Could you check a few things on this model? Use its own coordinates, in mm. A direction names the side the tool comes from. Give positions to 0.01 mm unless a question says otherwise; leave off trailing zeros. Write each loop counter-clockwise with the first axis right and the second up, starting at its lowest first coordinate (ties: lowest second). Pieces come first, ordered by that corner, then holes. Notation, with made-up numbers: (71.25, -21.75) -> (91.25, -21.75) arc R17 ccw to (91.25, 0.25) -> close; hole circle Ø8 at (33.25, 12.25). An arc over 180 degrees is marked (long way). Write item = value, one per line. Start each with the question number.
```python
from build123d import *

# Parameters (mm, degrees)
SKETCH_1_W             = 42
SKETCH_1_H             = 10
EXTRUDE_1_DEPTH        = 23.5
CUT_EXTRUDE_1_DEPTH    = 52.720402164
HOLE_WIZARD_M4_2_D     = 3.3
HOLE_WIZARD_M4_2_DEPTH = 10.1
HOLE_WIZARD_M4_2_TIP   = 0.991420021
HOLE_WIZARD_M4_1_D     = 3.3
CHAMFER_4_SIZE         = 12
CUT_EXTRUDE_3_DEPTH    = 34.064331336


with BuildPart() as part:
    # 草图1 → 凸台-拉伸1 (new, symmetric)
    with BuildSketch(Plane(origin=(0, 0, 0), x_dir=(0, 0, -1), z_dir=(1, 0, 0))):
        Rectangle(SKETCH_1_W, SKETCH_1_H)
    extrude(amount=EXTRUDE_1_DEPTH, both=True)

    # 草图2 → 切除-拉伸1 (cut, through all)
    with BuildSketch(Plane(origin=(23.5, 0, 0), x_dir=(0, 0, -1), z_dir=(1, 0, 0))):
        Polygon((21, -5), (11, 5), (21, 5), align=None)
    extrude(amount=-CUT_EXTRUDE_1_DEPTH, mode=Mode.SUBTRACT)

    # M4 螺纹孔2
    with Locations(Plane(origin=(-23.5, -27.863076326, 2.458563873), x_dir=(0, -1, 0), z_dir=(-1, 0, 0))):
        with Locations((-27.863076326, 5.541436127), (-27.863076326, -6.458563873)):
            Hole(HOLE_WIZARD_M4_2_D / 2, depth=HOLE_WIZARD_M4_2_DEPTH)
            with Locations((0, 0, -(HOLE_WIZARD_M4_2_DEPTH + HOLE_WIZARD_M4_2_TIP / 2))):  # 118° drill point
                Cone(0, HOLE_WIZARD_M4_2_D / 2, HOLE_WIZARD_M4_2_TIP, mode=Mode.SUBTRACT)

    # M4 螺纹孔1 (through all)
    with Locations(Plane(origin=(0, -5, 0), x_dir=(-1, 0, 0), z_dir=(0, -1, 0))):
        with Locations((-2.5, 17), (-17.222431864, -8.5), (12.222431864, -8.5)):
            Hole(HOLE_WIZARD_M4_1_D / 2)

    # 倒角4
    chamfer_4_edges = [part.edges().sort_by_distance(p)[0] for p in [
        (23.5, 0, 21),
    ]]
    chamfer(chamfer_4_edges, length=CHAMFER_4_SIZE)

    # 草图8 → 切除-拉伸3 (cut, through all)
    with BuildSketch(Plane.XZ.offset(5)):
        Polygon((23.5, -9), (11.5, -21), (23.5, -21), align=None)
    extrude(amount=-CUT_EXTRUDE_3_DEPTH, mode=Mode.SUBTRACT)


solid = part.part
```
(1) Imagine slicing it at C-C (y = -2.5). Please give me the cut outline in (x, z).
(2) On a 3-axis mill with a long thin cutter (end or side, diameter ignored), from which of +Z, -Z, +X, -X, +Y, -Y can I reach the whole of each face in a straight line? I mean faces 1 (the cylindrical face through (2.1, -2.7, -15.4)), 2 (the cylindrical face through (-18.379, -1.216, 9.115)). Say none if no direction works.
(3) I'm going to push flat-ended pins straight in: pin 1 (2 mm diameter, centred on x = 13, y = 2.5, fed in from -Z); pin 2 (4 mm diameter, centred on y = 2.5, z = -14.5, fed in from +X); pin 3 (5.5 mm diameter, centred on x = 2.5, z = -17, fed in from +Y); pin 4 (2 mm diameter, centred on x = -12.22, z = 8.5, fed in from +Y). Where does each tip first touch, or does it pass through?
(4) If I drill on line 1 along X through (y, z) = (3, 8.5); line 2 along Y through (x, z) = (-20.5, -4); line 3 along Z through (x, y) = (-20, 0), over which ranges is the centre line in solid material (lowest first)? Write a range as from..to.
(5) Imagine slicing it at B-B (z = -17). Please give me the cut outline in (x, y), then the cut area to 3 significant figures.
(6) Imagine slicing it at A-A (x = 2.5). Please give me the cut outline in (y, z).
(7) We'd pull the mould along Z, two halves only. Please class faces 3 (the cylindrical face through (-18.4, -0.4, -5.6)), 4 (the flat face through (18.9, -1.2, -13.6)), 5 (the flat face through (23.5, 0, 0)), 6 (the cylindrical face through (-10.698, 0.07, 9.132)): released by +Z, released by -Z, zero draft, split by the parting line, or undercut.
(8) Imagine slicing it at D-D (z = 16). Please give me the cut outline in (x, y), then the cut area to 3 significant figures.
Answers below:
q1.outline = (-23.5, -18.5) -> (1.81, -18.5) arc R1.65 cw (long way) to (3.19, -18.5) -> (14, -18.5) -> (23.5, -9) -> (23.5, 9) -> (11.5, 21) -> (-23.5, 21) -> close; hole circle Ø3.3 at (-12.22, 8.5); hole circle Ø3.3 at (17.22, 8.5)
q2.face_1 = +Y, -Y
q2.face_2 = -X
q3.pin_1 = -14.5
q3.pin_2 = 20
q3.pin_3 = 1.75
q3.pin_4 = through
q4.line_1 = -23.5..-13.87, -10.57..15.57, 18.87..23.5
q4.line_2 = -5..-1.65, 1.65..5
q4.line_3 = -16..-5.65, -2.35..6.35, 9.65..21
q5.outline = (-23.5, -5) -> (0.85, -5) -> (0.85, -1) -> (-23.5, -1) -> close; (4.15, -5) -> (15.5, -5) -> (15.5, -1) -> (4.15, -1) -> close
q5.area = 143 mm^2
q6.outline = (-5, -21) -> (-2.65, -18.65) -> (-5, -18.65) -> close; (-5, -15.35) -> (0.65, -15.35) -> (5, -11) -> (5, 21) -> (-5, 21) -> close
q7.face_3 = undercut
q7.face_4 = released by -Z
q7.face_5 = zero draft
q7.face_6 = undercut
q8.outline = (-23.5, -5) -> (16.5, -5) -> (16.5, 5) -> (-23.5, 5) -> close
q8.area = 400 mm^2
